The figure shows three views and two pictorial views of one solid part (mm, origin at its lowest corner). Answer the questions. A direction names the side the tool comes from. Coordinates: 2 decimals unless noted, no trailing zeros. Order: outer loops, then holes, each group sorted by start corner. A loop starts at its lowest first (then second) coordinate and runs counter-clockwise, first axis right, second up. Notation, with made-up numbers: (-20.75, -7) -> (-7.75, -7) arc R18 ccw to (-7.75, 27) -> close; hole circle Ø8 at (25.25, 5.25). An arc over 180 degrees is marked (long way). Return JSON: item names as keys, results as strings. Group by question number.
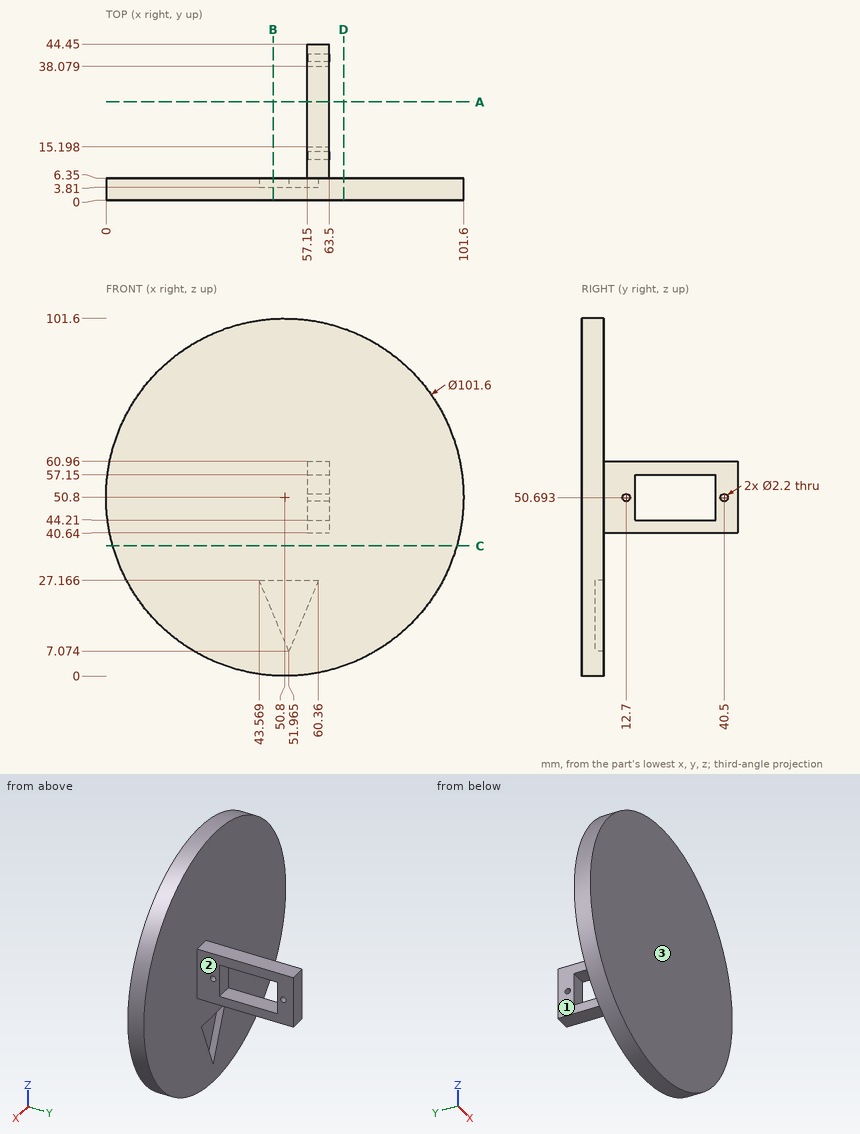
1. Find section C-C on z = 37. Determine the outline of the cut face in (x, y).
2. Find section A-A on y = 28. Determine the outline of the cut face in (x, z).
3. Straight lines are drawn through the part: L1, parallel to Y at x = 6, z = 62; L2, parallel to X at y = 23.5, z = 60.5; L3, parallel to Z at x = 58, y = 40. For each, find the intervals that lie inside material, in ascending order.
4. Find section D-D on x = 67.5. Determine the outline of the cut face in (y, z), and give its area (3 significant figures).
5. Find section B-B on x = 47.5. Determine the outline of the cut face in (y, z), and give its area (3 significant figures).
6. Which of the six approach directions +Z, -Z, +X, -X, +Y, -Y give full straight-line access (tool end or side, diameter ignored) to the marked faces 1, 2 and 3?
7. Given pin 1 (1.9 mm diameter, centred on x = 62, y = 23.5, fed in from -Z); pin 2 (12 mm diameter, centred on x = 90.5, z = 39, fed in from +Y); pin 3 (1.3 mm diameter, centred on y = 40.5, z = 50.69, fed in from +X) (1 decimal); pin 4 (16.5 mm diameter, centred on y = 17, z = 54, fed in from +X), each flat-ended and moving along its own axis, determine where each tip first touches the part or whether it passes through.
Result:
{
 "1": {"outline": "(1.91, 0) -> (99.69, 0) -> (99.69, 6.35) -> (1.91, 6.35) -> close"},
 "2": {"outline": "(57.15, 40.64) -> (63.5, 40.64) -> (63.5, 44.21) -> (57.15, 44.21) -> close; (57.15, 57.15) -> (63.5, 57.15) -> (63.5, 60.96) -> (57.15, 60.96) -> close"},
 "3": {"L1": "0 to 6.35", "L2": "57.15 to 63.5", "L3": "40.64 to 49.71, 51.67 to 60.96"},
 "4": {"outline": "(0, 2.82) -> (6.35, 2.82) -> (6.35, 98.78) -> (0, 98.78) -> close", "area": "609 mm^2"},
 "5": {"outline": "(0, 0.11) -> (6.35, 0.11) -> (6.35, 17.76) -> (3.81, 17.76) -> (3.81, 27.17) -> (6.35, 27.17) -> (6.35, 101.49) -> (0, 101.49) -> close", "area": "620 mm^2"},
 "6": {"face 1": "+Z, -Z, -X, +Y", "face 2": "+Z, -Z, +X, +Y", "face 3": "+Z, -Z, +X, -X, -Y"},
 "7": {"pin 1": "z = 40.64", "pin 2": "y = 6.35", "pin 3": "through", "pin 4": "x = 63.5"}
}
